Geometry: final body of the model. Coordinates: model frame, mm. Give positions to 0.01 mm unless a question says otherwise; leave off trailing zeros. Loops run counter-clockwise (first coordinate to the right, second up) from the corner with the lowest first, then second, coordinate; pieces in that order, holes last. Notation, with made-up numbers: (63.25, 43) - (73.25, 43) arc R10 cw to (73.25, 53) - close; hole circle Ø6 at (-30.75, 57.5). An arc over 180 degrees is marked (long way). Answer in a Markdown table with one row per item.
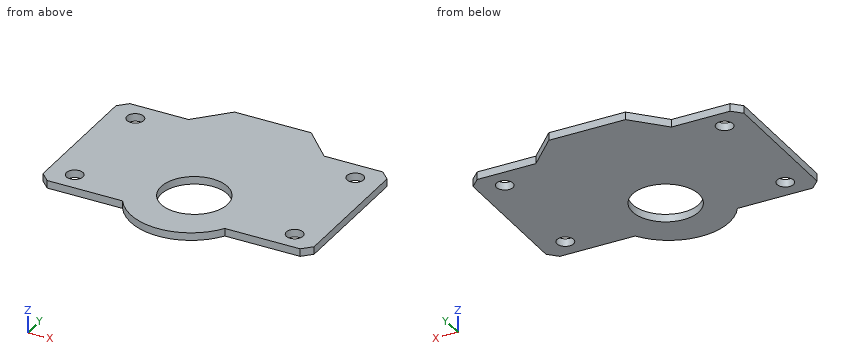
from build123d import *

# Parameters (mm, degrees)
F1_DEPTH = 3
F2_R     = 13
F3_DEPTH = 3.001
F4_R     = 3.25
F5_DEPTH = 3.001


with BuildPart() as f1:
    # F0 (on Top) → F1 (new body)
    with BuildSketch(Plane.XY):
        with BuildLine():
            Line((-26.5, 30), (-49.464466, 30))
            Line((-49.464466, 30), (-53, 26.464466))
            Line((-53, 26.464466), (-53, -26.464466))
            Line((-53, -26.464466), (-49.464466, -30))
            Line((-49.464466, -30), (-20, -30))
            ThreePointArc((-20, -30), (0, -41), (20, -30))
            Line((20, -30), (49.464466, -30))
            Line((49.464466, -30), (53, -26.464466))
            Line((53, -26.464466), (53, 26.464466))
            Line((53, 26.464466), (49.464466, 30))
            Line((49.464466, 30), (26.5, 30))
            Line((26.5, 30), (15, 42))
            Line((15, 42), (-15, 42))
            Line((-15, 42), (-26.5, 30))
        make_face()
    extrude(amount=F1_DEPTH)

    # F2 (on face) → F3 (cut, through all)
    with BuildSketch(Plane.XY.offset(3)):
        with Locations((0, -15)):
            Circle(F2_R)
    extrude(amount=-F3_DEPTH, mode=Mode.SUBTRACT)

    # F4 (on face) → F5 (cut, through all)
    with BuildSketch(Plane.XY.offset(3)):
        with Locations((-43, 22)):
            Circle(F4_R)
        with Locations((-43, -22)):
            Circle(F4_R)
        with Locations((43, 22)):
            Circle(F4_R)
        with Locations((43, -22)):
            Circle(F4_R)
    extrude(amount=-F5_DEPTH, mode=Mode.SUBTRACT)


solid = f1.part
Q1. Cut plane A-A (y = -15). Output: boundary loops of the cut face in (x, z).
Check values:
| item | result |
|---|---|
| outline | (-53, 0) - (-13, 0) - (-13, 3) - (-53, 3) - close; (13, 0) - (53, 0) - (53, 3) - (13, 3) - close |
Q2. First-contact query: pin 1 (10.5 mm diameter, centred on x = -43, y = -22, fed in from +Z); pin 2 (3 mm diameter, centred on x = -40.5, y = 32, fed in from -Z); pin 3 (1.5 mm diameter, centred on x = 42.5, z = 2, fed in from +Y). Flat tips, straight axial feed; report the tip coordinate or a pass-through.
Check values:
| item | result |
|---|---|
| pin 1 | z = 3 |
| pin 2 | through |
| pin 3 | y = 30 |
Q3. Cut plane C-C (y = 22). Output: boundary loops of the cut face in (x, z).
Check values:
| item | result |
|---|---|
| outline | (-53, 0) - (-46.25, 0) - (-46.25, 3) - (-53, 3) - close; (-39.75, 0) - (39.75, 0) - (39.75, 3) - (-39.75, 3) - close; (46.25, 0) - (53, 0) - (53, 3) - (46.25, 3) - close |
Q4. Material intervals for line 1 along Y through (x, z) = (43, 1.65); line 2 along X through (y, z) = (-3.5, 1.4); line 3 along Y through (x, z) = (-29.5, 2.75), sorted ascending.
Check values:
| item | result |
|---|---|
| line 1 | -30 to -25.25, -18.75 to 18.75, 25.25 to 30 |
| line 2 | -53 to -6.06, 6.06 to 53 |
| line 3 | -30 to 30 |
Q5. Cut plane D-D (x = -3.5). Output: boundary loops of the cut face in (y, z), and give its area (3 significant figures).
Check values:
| item | result |
|---|---|
| outline | (-40.74, 0) - (-27.52, 0) - (-27.52, 3) - (-40.74, 3) - close; (-2.48, 0) - (42, 0) - (42, 3) - (-2.48, 3) - close |
| area | 173 mm² |
Q6. Cut plane B-B (x = 43). Output: boundary loops of the cut face in (y, z).
Check values:
| item | result |
|---|---|
| outline | (-30, 0) - (-25.25, 0) - (-25.25, 3) - (-30, 3) - close; (-18.75, 0) - (18.75, 0) - (18.75, 3) - (-18.75, 3) - close; (25.25, 0) - (30, 0) - (30, 3) - (25.25, 3) - close |
